Geometry: final body of the model. Coordinates: model frame, mm. Face numbers are marked on the shaded views. A direction names the side the tool comes from. Give positions to 0.01 mm unless a question says otherwise; leave off trailing zeros. Write each loop counter-clockwise with the first axis right and the second up, starting at its lowest first coordinate (ties: lowest second). Pieces come first, ordered by that corner, then holes. Notation, with made-up numbers: (13.25, -2.5) - (54.25, -2.5) arc R30 ccw to (54.25, 29.5) - close; hole circle Ø4 at (23, 4.5). An arc over 180 degrees is marked (long way). Use CSV: the item, a comma, the result in double quotes. Start each with the question number.
(1) First-contact query: pin 1 Ø12.5 at (y, z) = (-9, 69) entering from -X; pin 2 Ø4 at (x, z) = (-45, 81.5) entering from -Y; pin 3 Ø5 at (x, z) = (-21.5, 76) entering from -Y. Flat tips, straight axial feed; report the tip coordinate or a pass-through.
(2) Section D-D on x = -26.5. Output: boundary loops of the cut face in (y, z).
(3) Line query: probe 1 along X at (y, z) = (12.9, 66); probe 2 along X at (y, z) = (-7.5, 74); probe 3 along X at (y, z) = (-10, 83.5). Output: solid intervals per line, ascending. Write a range as [from, to].
(4) Reachability of the marked faces 1, 2 and 3 from +Z, -Z, +X, -X, +Y, -Y: full face, straight path, thin tool, end or side. Return the list, or none.
(5) Section B-B on y = 0.5. Output: boundary loops of the cut face in (x, z), and give its area (3 significant figures).
(6) Draft query along X for the marked faces 4, 5, 6 and 7. Return one class per face: released by +X, released by -X, zero draft, split by the parting line, or undercut.
(7) Section C-C on z = 84. Count the separate pieces of the cut face and the enclosed holes in it, and give its area (3 significant figures).
(8) Section A-A on x = -55.6. Output: boundary loops of the cut face in (y, z), and give its area (3 significant figures).
from build123d import *

# Parameters (mm, degrees)
EXTRUDE1_DEPTH      = 20
EXTRUDE1_DEPTH_BACK = 10
SKETCH2_W           = 22.028427124
SKETCH2_H           = 1.9
SKETCH3_R           = 1.6
CUT_EXTRUDE1_DEPTH  = 20
SKETCH4_R           = 2.15
CUT_EXTRUDE2_DEPTH  = 15


with BuildPart() as part:
    # Sketch2 → Extrude1 (new, two sides: drawn at the far end of the back side and taken through both)
    with BuildSketch(Plane.XY.offset(70).offset(-EXTRUDE1_DEPTH_BACK)):
        Polygon((31.6, 1.959185913), (31.6, -13.690519995), (12.781818432, -17.14052), (-12.781818445, -17.14052), (-31.6, -13.690519995), (-31.6, -8.571067812), (-45.6, -8.571067812), (-45.6, -11.571067812), (-35.6, -11.571067812), (-35.6, -17.023853319), (-13.145454814, -21.14052), (13.145454801, -21.14052), (35.6, -17.023853319), (35.6, 3.428932188), (42.671067812, 10.5), (65.6, 10.5), (65.6, 14.5), (-65.6, 14.5), (-65.6, 10.5), (-42.671067812, 10.5), (-35.6, 3.428932188), (-35.6, -4.571067812), (-45.6, -4.571067812), (-45.6, -7.571067812), (-31.6, -7.571067812), (-31.6, 1.959185913), (-9.945324486, 4.6), (9.945324486, 4.6), align=None)
        Polygon((37.014213562, 10.5), (32.404878042, 5.890664479), (15.014213562, 8.011477221), (15.014213562, 10.5), align=None, mode=Mode.SUBTRACT)
        with Locations((0, 9.55)):
            Rectangle(SKETCH2_W, SKETCH2_H, mode=Mode.SUBTRACT)
        Polygon((-15.014213562, 10.5), (-15.014213562, 8.011477221), (-32.404878042, 5.890664479), (-37.014213562, 10.5), align=None, mode=Mode.SUBTRACT)
    extrude(amount=EXTRUDE1_DEPTH + EXTRUDE1_DEPTH_BACK)

    # Sketch3 → Cut-Extrude1 (cut)
    with BuildSketch(Plane.XZ.offset(-10.5)):
        with Locations((-55.6, 84)):
            Circle(SKETCH3_R)
        with Locations((-55.6, 66)):
            Circle(SKETCH3_R)
        with Locations((55.6, 84)):
            Circle(SKETCH3_R)
        with Locations((55.6, 66)):
            Circle(SKETCH3_R)
    extrude(amount=-CUT_EXTRUDE1_DEPTH, mode=Mode.SUBTRACT)

    # Sketch4 → Cut-Extrude2 (cut)
    with BuildSketch(Plane.XZ.offset(11.571067812)):
        with Locations(Location((-41.6, 75, 0), (0, 0, 270))):
            Circle(SKETCH4_R)
    extrude(amount=-CUT_EXTRUDE2_DEPTH, mode=Mode.SUBTRACT)


solid = part.part
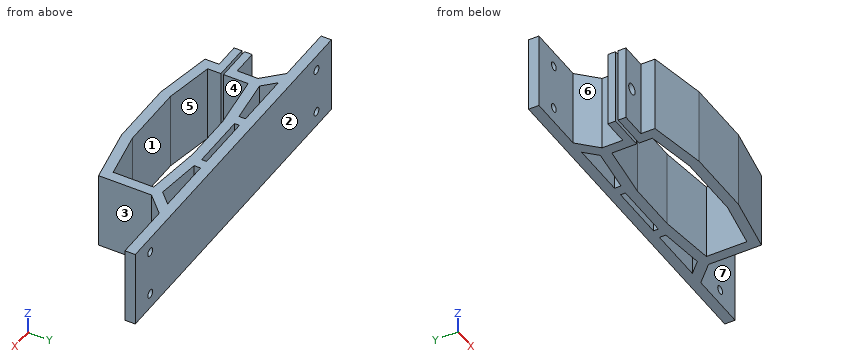
Check values:
1,pin 1,"stops at x = -45.6"
1,pin 2,"stops at y = -11.57"
1,pin 3,"stops at y = -20.07"
2,outline,"(-18.69, 60) - (-14.63, 60) - (-14.63, 90) - (-18.69, 90) - close; (2.58, 60) - (6.61, 60) - (6.61, 90) - (2.58, 90) - close; (10.5, 60) - (14.5, 60) - (14.5, 90) - (10.5, 90) - close"
3,probe 1,"x = [-65.6, -57.2], [-54, 54], [57.2, 65.6]"
3,probe 2,"x = [-45.6, -43.5], [-39.7, -31.6], [31.6, 35.6]"
3,probe 3,"x = [-45.6, -31.6], [31.6, 35.6]"
4,face 1,"+Z, -Z"
4,face 2,"+Z, -Z, +X, -X, +Y"
4,face 3,"+Z, -Z, +X, -Y"
5,outline,"(-35.6, 60) - (-31.6, 60) - (-31.6, 90) - (-35.6, 90) - close; (31.6, 60) - (35.6, 60) - (35.6, 90) - (31.6, 90) - close"
5,area,"240 mm²"
6,face 4,"undercut"
6,face 5,"undercut"
6,face 6,"released by -X"
6,face 7,"zero draft"
7,separate pieces,"3"
7,enclosed holes,"3"
7,area,"1,330 mm²"
8,outline,"(10.5, 60) - (14.5, 60) - (14.5, 64.4) - (10.5, 64.4) - close; (10.5, 67.6) - (14.5, 67.6) - (14.5, 82.4) - (10.5, 82.4) - close; (10.5, 85.6) - (14.5, 85.6) - (14.5, 90) - (10.5, 90) - close"
8,area,"94.4 mm²"
